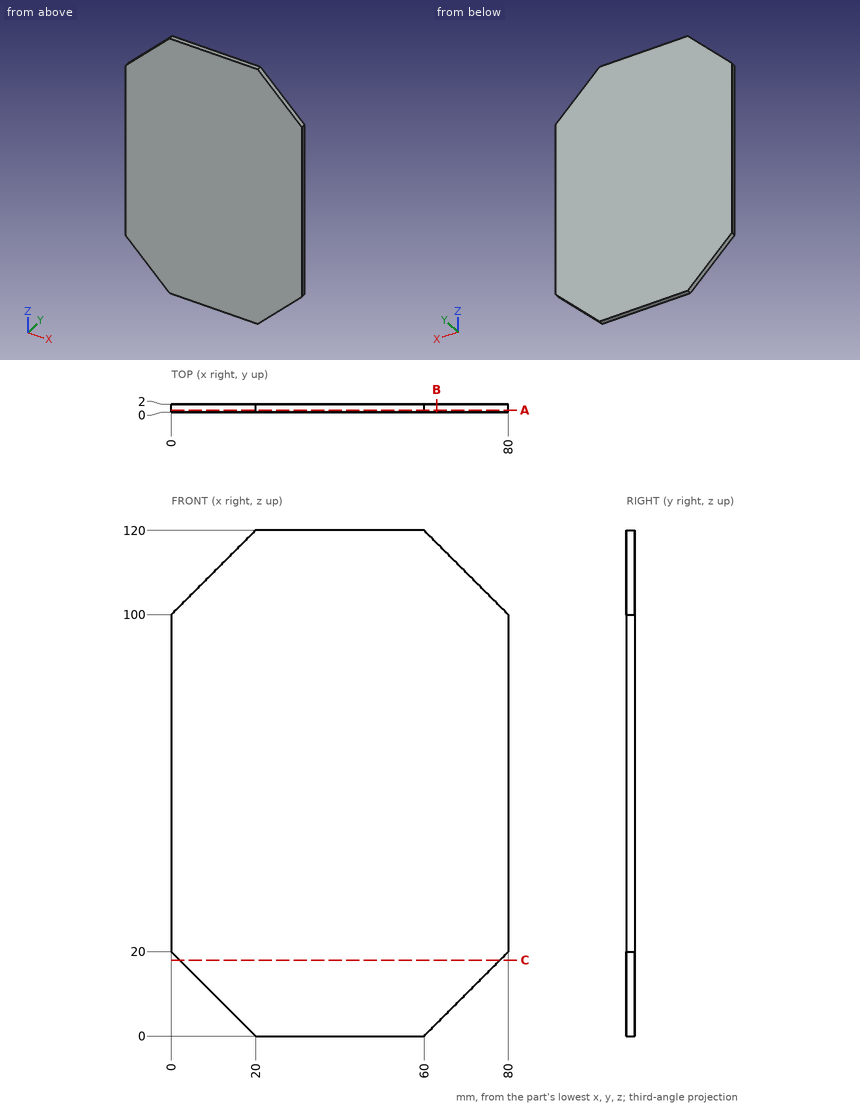
Study the drawing (mm; zero at the part's minimum x, y, z) and answer. Round coordinates to 2 decimals unless told otherwise and drop trailing zeros. Loops run counter-clockwise (first coordinate to the right, second up) from the corner with the lowest first, then second, coordinate; pieces in that order, holes last. Notation, with made-up numbers: M -22,-38.75 L -8,-38.75 A6 ccw -8,-32.75 Z; hole C -28,-14 d11. An arc over 180 degrees is marked long. One line per question, with ' | ' between items.
Q1. Find section C-C, the plane z = 18. Give the vertices of the cut face in (x, y), then the cut area to 3 significant figures.
Conclusion:
outline: M 2,0 L 78,0 L 78,2 L 2,2 Z | area: 152 mm2
Q2. Consider line 1 along X through (y, z) = (1.9, 107); line 2 along Z through (x, y) = (77.5, 0.65); line 3 along X through (y, z) = (1.5, 102.5). Determine where each line is inside the solid, lowest interval first. Write a range as from..to.
Conclusion:
line 1: x = 7..73 | line 2: z = 17.5..102.5 | line 3: x = 2.5..77.5
Q3. Find section B-B, the plane x = 63. Give the vertices of the cut face in (y, z).
Conclusion:
outline: M 0,3 L 2,3 L 2,117 L 0,117 Z
Q4. Find section A-A, the plane y = 0.55. Give the vertices of the cut face in (x, z), then the cut area to 3 significant figures.
Conclusion:
outline: M 0,20 L 20,0 L 60,0 L 80,20 L 80,100 L 60,120 L 20,120 L 0,100 Z | area: 8,800 mm2
Q5. This flat-tipped pin is pushed along its axis until it touches: pin 1 Ø5 at (x, z) = (35.5, 99.5) entering from -Y. Where does it stop, or does it pass through?
Conclusion:
pin 1: stops at y = 0
